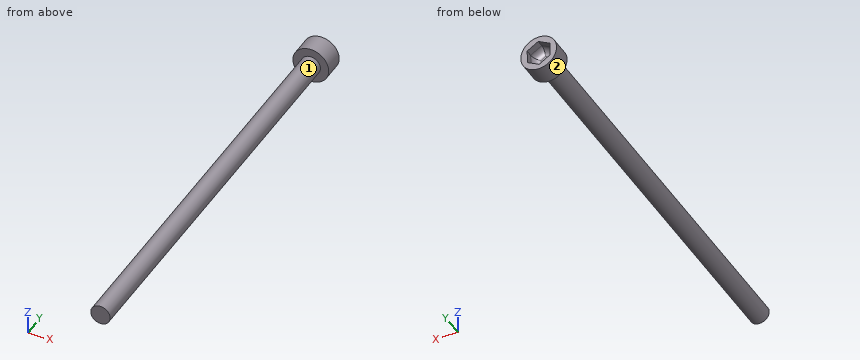
```python
from build123d import *

# Parameters (mm, degrees)
CUT_EXTRUDE1_DEPTH = 2
FILLET1_R          = 1


with BuildPart() as part:
    # Sketch1 → Revolve2 (revolve)
    with BuildSketch(Plane.XY):
        Polygon((0, 0), (1.44, 0), (1.44, 60), (2.665, 60), (2.665, 63), (0, 63), align=None)
    revolve(axis=Axis((0, 0, 0), (0, 1, 0)))

    # Sketch3 → Cut-Extrude1 (cut)
    with BuildSketch(Plane(origin=(0, 63, 0), x_dir=(1, 0, 0), z_dir=(0, 1, 0))):
        Polygon((1.720029198, -0.914625258), (1.652103308, 1.032276352), (-0.067925891, 1.94690161), (-1.720029198, 0.914625258), (-1.652103308, -1.032276352), (0.067925891, -1.94690161), align=None)
    extrude(amount=-CUT_EXTRUDE1_DEPTH, mode=Mode.SUBTRACT)

    # Fillet1
    fillet1_edges = [part.edges().sort_by_distance(p)[0] for p in [
        (0.893977545, 61, 1.430763434),
        (-0.792088708, 61, 1.489588981),
        (-1.686066253, 61, 0.058825547),
        (-0.893977545, 61, -1.430763434),
        (0.792088708, 61, -1.489588981),
        (1.686066253, 61, -0.058825547),
    ]]
    fillet(fillet1_edges, radius=FILLET1_R)


solid = part.part
```
Check sheet for the modelled part. Datum: model origin and axes. Units: mm. Face numbers are marked on the shaded views. A direction names the side the tool comes from. Give positions to 0.01 mm unless a question says otherwise; leave off trailing zeros. Order: outer loops, then holes, each group sorted by start corner. A loop starts at its lowest first (then second) coordinate and runs counter-clockwise, first axis right, second up. Notation, with made-up numbers: M -35.5,10.25 L -14.5,10.25 A32 cw -14.5,38.25 Z; hole C 86.5,-11 d11. An arc over 180 degrees is marked long. Answer in a Markdown table with one row per item. Add a question column.
Q1. Access from +Z, -Z, +X, -X, +Y, -Y to the whole of each face (thin tool, end or side, straight path). Record for the marked faces 1 and 2.
Q2. Thickness scan on L1, parallel to Y at x = -0.6, z = 1.65; L2, parallel to X at y = 33.5, z = 1; L3, parallel to Y at x = 0.5, z = 0.5. Record the ranges inside material, lowest first.
Q3. Gauge pin test, flat ends, axial feed: pin 1 Ø1 at (x, y) = (0.5, 42.5) entering from -Z; pin 2 Ø1 at (y, z) = (34, 1) entering from -X; pin 3 Ø2 at (y, z) = (8.5, 1.5) entering from +X; pin 4 Ø1.6 at (x, z) = (-1, -1) entering from -Y. Record the tip position at first contact, or that the pin passes through.
Q4. Sectioned sample at A-A, the plane y = 30. Record the boundary of the cut face in (x, z), and give its area (3 significant figures).
Verdict:
| question | item | result |
|---|---|---|
| 1 | face 1 | -Y |
| 1 | face 2 | +Y, -Y |
| 2 | L1 | 60 to 63 |
| 2 | L2 | -1.04 to 1.04 |
| 2 | L3 | 0 to 61 |
| 3 | pin 1 | z = -1.44 |
| 3 | pin 2 | x = -1.35 |
| 3 | pin 3 | x = 1.35 |
| 3 | pin 4 | y = 0 |
| 4 | outline | C 0,0 d2.88 |
| 4 | area | 6.51 mm² |
